Verification items for the finished model (mm, model axes). Face numbers are marked on the shaded views. A direction names the side the tool comes from. Round coordinates to 2 decimals unless told otherwise and drop trailing zeros. Order: outer loops, then holes, each group sorted by start corner. A loop starts at its lowest first (then second) coordinate and runs counter-clockwise, first axis right, second up. Notation, with made-up numbers: (80, 22.25) -> (127, 22.25) arc R19 ccw to (127, 45.25) -> close; hole circle Ø2 at (83, 0). An arc over 180 degrees is marked (long way). Return JSON: item names as keys, results as strings. Group by question number.
Item 1: Scan lines: probe 1 along Y at (x, z) = (1.25, -30); probe 2 along X at (y, z) = (16.5, -32). Record each from-to range of solid material in increasing order. Write a range as from..to.
Item 2: Sectioned sample at C-C on x = 2.25. Record the cut outline in (y, z), plus the area to 3 significant figures.
Item 3: Depth check by flat-ended pin: pin 1 Ø6 at (x, z) = (6, -11) entering from +Y; pin 2 Ø1.5 at (x, y) = (3, -4) entering from +Z; pin 3 Ø10 at (y, z) = (-1.5, -23) entering from -X; pin 4 Ø3.5 at (y, z) = (-10, -30) entering from -X (3 decimals). Enter the tip coordinate at first touch or a pass-through.
Item 4: Sectioned sample at D-D on z = -18.5. Record the cut outline in (x, y), plus the area to 3 significant figures.
Item 5: Access from +Z, -Z, +X, -X, +Y, -Y to the whole of each face (thin tool, end or side, straight path). Record for the marked faces 1, 2, 3 and 4.
Item 6: Sectioned sample at A-A on z = -30. Record the cut outline in (x, y), plus the area to 3 significant figures.
Item 7: Sectioned sample at B-B on y = -10. Record the cut outline in (x, z).
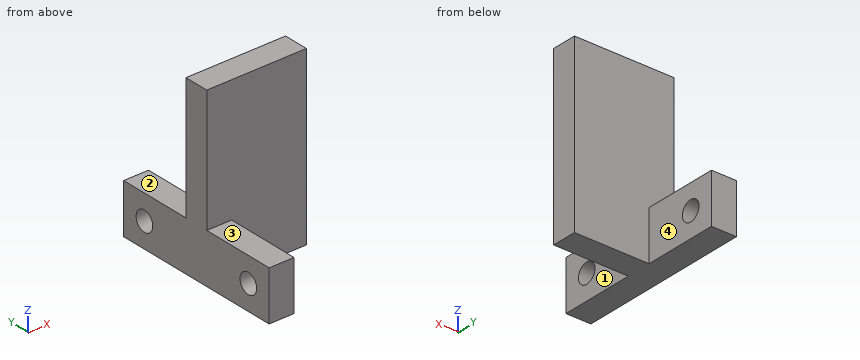
```python
from build123d import *

# Parameters (mm, degrees)
SKETCH1_W           = 35
SKETCH1_H           = 5
BOSS_EXTRUDE1_DEPTH = 20
SKETCH2_W           = 5
SKETCH2_H           = 10
BOSS_EXTRUDE2_DEPTH = 15
SKETCH3_W           = 5
SKETCH3_H           = 10
BOSS_EXTRUDE3_DEPTH = 15
SKETCH4_R           = 2
CUT_EXTRUDE1_DEPTH  = 15


with BuildPart() as part:
    # Sketch1 → Boss-Extrude1 (new body)
    with BuildSketch(Plane(origin=(0, 0, 0), x_dir=(0, 0, -1), z_dir=(1, 0, 0))):
        with Locations((17.5, 2.5)):
            Rectangle(SKETCH1_W, SKETCH1_H)
    extrude(amount=BOSS_EXTRUDE1_DEPTH)

    # Sketch2 → Boss-Extrude2 (add)
    with BuildSketch(Plane(origin=(0, 5, 0), x_dir=(1, 0, 0), z_dir=(0, 1, 0))):
        with Locations((2.5, 30)):
            Rectangle(SKETCH2_W, SKETCH2_H)
    extrude(amount=BOSS_EXTRUDE2_DEPTH)

    # Sketch3 → Boss-Extrude3 (add)
    with BuildSketch(Plane.XZ):
        with Locations((2.5, -30)):
            Rectangle(SKETCH3_W, SKETCH3_H)
    extrude(amount=BOSS_EXTRUDE3_DEPTH)

    # Sketch4 → Cut-Extrude1 (cut)
    with BuildSketch(Plane(origin=(5, 0, 0), x_dir=(0, 0, -1), z_dir=(1, 0, 0))):
        with Locations((30, 15)):
            Circle(SKETCH4_R)
        with Locations((30, -10)):
            Circle(SKETCH4_R)
    extrude(amount=-CUT_EXTRUDE1_DEPTH, mode=Mode.SUBTRACT)


solid = part.part
```
Recorded:
{
 "1": {"probe 1": "-15..-12, -8..13, 17..20", "probe 2": "0..5"},
 "2": {"outline": "(-15, -35) -> (20, -35) -> (20, -25) -> (5, -25) -> (5, 0) -> (0, 0) -> (0, -25) -> (-15, -25) -> close; hole circle Ø4 at (-10, -30); hole circle Ø4 at (15, -30)", "area": "450 mm²"},
 "3": {"pin 1": "y = 5", "pin 2": "z = -25", "pin 3": "x = 0", "pin 4": "through"},
 "4": {"outline": "(0, 0) -> (20, 0) -> (20, 5) -> (0, 5) -> close", "area": "100 mm²"},
 "5": {"face 1": "+Z, -Z, +X, -Y", "face 2": "+Z, +X, -X, +Y", "face 3": "+Z, +X, -X, -Y", "face 4": "+Z, -Z, +X, +Y"},
 "6": {"outline": "(0, -15) -> (5, -15) -> (5, -12) -> (0, -12) -> close; (0, -8) -> (5, -8) -> (5, 0) -> (20, 0) -> (20, 5) -> (5, 5) -> (5, 13) -> (0, 13) -> close; (0, 17) -> (5, 17) -> (5, 20) -> (0, 20) -> close", "area": "210 mm²"},
 "7": {"outline": "(0, -35) -> (5, -35) -> (5, -32) -> (0, -32) -> close; (0, -28) -> (5, -28) -> (5, -25) -> (0, -25) -> close"}
}
